Autodesk Inventor part; units mm, degrees
ref_plane "YZ Plane" through (0, 0, 0) normal (1, 0, 0) x (0, 1, 0)
ref_plane "XZ Plane" through (0, 0, 0) normal (0, 1, 0) x (-1, 0, 0)
ref_plane "XY Plane" through (0, 0, 0) normal (0, 0, 1) x (1, 0, 0)
sketch "Sketch1" plane through (0, 0, 0) normal (0, 0, 1) x (1, 0, 0)
  line L0 (147.6375, 0) -> (-128.5875, 0)
  line L1 (-128.5875, 0) -> (-128.5875, 917.575)
  line L2 (-128.5875, 917.575) -> (147.6375, 917.575)
  line L3 (147.6375, 917.575) -> (147.6375, 0)
  line L4 (142.875, 912.8125) -> (-123.825, 912.8125)
  line L5 (-123.825, 912.8125) -> (-123.825, 4.7625)
  line L6 (-123.825, 4.7625) -> (142.875, 4.7625)
  line L7 (142.875, 4.7625) -> (142.875, 912.8125)
  point P0 (0, 0)
extrude "Extrusion1" add sketch "Sketch1" against normal blind 281.94
properties part number "uv environment" material "PMMA Plastic"
Design review of the part built by this model. Coordinates are the model's own, in mm. A direction names the side the tool comes from. Coordinates: 2 decimals unless noted, no trailing zeros. Loops run counter-clockwise (first coordinate to the right, second up) from the corner with the lowest first, then second, coordinate; pieces in that order, holes last. Notation, with made-up numbers: (12.25, -12) - (53.25, -12) arc R37 cw to (53.25, 26) - close; hole circle Ø8 at (37.25, 85). An arc over 180 degrees is marked (long way). Use CSV: the item, a comma, the result in double quotes. Start each with the question number.
1) Wall thickness on L1, parallel to Y at x = 81, z = -261 (1 decimal); L2, parallel to X at y = 795, z = -229 (1 decimal): over which ranges is each line inside the solid? List them lowest first. Write a range as from..to.
2) Consider section A-A on x = -81.5. Write out the cut boundary in (y, z) (1 decimal).
3) The part is to be moulded in two halves that separate along Y. For faces 1 (the flat face through (11, 0, -139)), 2 (the flat face through (8, 4.762, -139)), 3 (the flat face through (-124, 461, 0)), say which applies: +Y half, -Y half, draft (parallel to the pull), parting line (faces both ways), or undercut.
4) Tool access review of faces 4 (the flat face through (147.638, 465, -139)), 5 (the flat face through (11, 912.812, -139)): name each direction out of +Z, -Z, +X, -X, +Y, -Y from which nothing blocks a thin tool from reaching the whole face with its end or side.
5) Consider section B-B on z = -33. Write out the cut boundary in (x, y) (1 decimal).
6) Consider section C-C on y = 489. Write out the cut boundary in (x, z) (1 decimal).
Geometry says:
1,L1,"0..4.8, 912.8..917.6"
1,L2,"-128.6..-123.8, 142.9..147.6"
2,outline,"(0, -281.9) - (4.8, -281.9) - (4.8, 0) - (0, 0) - close; (912.8, -281.9) - (917.6, -281.9) - (917.6, 0) - (912.8, 0) - close"
3,face 1,"-Y half"
3,face 2,"undercut"
3,face 3,"draft"
4,face 4,"+Z, -Z, +X, +Y, -Y"
4,face 5,"+Z, -Z"
5,outline,"(-128.6, 0) - (147.6, 0) - (147.6, 917.6) - (-128.6, 917.6) - close; hole (-123.8, 4.8) - (142.9, 4.8) - (142.9, 912.8) - (-123.8, 912.8) - close"
6,outline,"(-128.6, -281.9) - (-123.8, -281.9) - (-123.8, 0) - (-128.6, 0) - close; (142.9, -281.9) - (147.6, -281.9) - (147.6, 0) - (142.9, 0) - close"
